Build history of the part. All positions in model axes, mm. A direction names the side the tool comes from. Round coordinates to 2 decimals unless told otherwise and drop trailing zeros. Loops run counter-clockwise (first coordinate to the right, second up) from the corner with the lowest first, then second, coordinate; pieces in that order, holes last. Notation, with made-up numbers: (41, -8) - (45, -8) arc R23 cw to (45, 10) - close; hole circle Ø3 at (-26, 75.25). An arc over 180 degrees is marked (long way). Use one line per item in the form item = value. Start each with the question number.
Q1. Drill centre lines: line 1 (Y direction, x = 0, z = 6); line 2 (Y direction, x = 28, z = 2.5); line 3 (Y direction, x = 4.5, z = 9.25). Where is each one in solid material? Low to high.
Q2. Saw through at C-C (z = 4). Count the separate pieces of the cut face and the enclosed holes in it, then the cut area to 3 significant figures.
Q3. Mould opens along X. For faces 3 (the face through (-27.44, 26.27, 5.07)), 4 (the face through (47.69, 15.02, 4.93)), 5 (the face through (9, -17, 10)) say: released by +X, released by -X, zero draft, split by the parting line, or undercut.
Q4. 3-axis set-ups, long thin cutter, end or side, ignore diameter. For faces 1 (the face through (-7, -20, 8)), 2 (the face through (8.767, -16.856, 4.93)): which of +Z, -Z, +X, -X, +Y, -Y reach the whole face in a straight line?
Q5. Saw through at A-A (x = 0). Give the cut face in (y, z).
Q6. Pin check, flat tips, straight feed: pin 1 (1 mm diameter, centred on x = -21, z = 2.5, fed in from -Y); pin 2 (2 mm diameter, centred on y = -24.5, z = 2, fed in from -X); pin 3 (2 mm diameter, centred on x = 15.5, z = 1, fed in from -Y). Stop position of each tip, or through.
Q7. Saw through at D-D (x = -23). Give the cut face in (y, z).
```python
from build123d import *

# Parameters (mm, degrees)
CROQUIS1_R              = 50
CROQUIS1_R_2            = 19
SALIENTE_EXTRUIR1_DEPTH = 10
CROQUIS4_R              = 30
CROQUIS4_R_2            = 20.75
CORTAR_EXTRUIR1_DEPTH   = 2
CROQUIS5_R              = 2.75
CORTAR_EXTRUIR2_DEPTH   = 10


with BuildPart() as part:
    # Croquis1 → Saliente-Extruir1 (new body)
    with BuildSketch(Plane.XY):
        Circle(CROQUIS1_R)
        Circle(CROQUIS1_R_2, mode=Mode.SUBTRACT)
    extrude(amount=SALIENTE_EXTRUIR1_DEPTH)

    # Croquis4 → Cortar-Extruir1 (cut)
    with BuildSketch(Plane.XY.offset(10)):
        Circle(CROQUIS4_R)
        Circle(CROQUIS4_R_2, mode=Mode.SUBTRACT)
    extrude(amount=-CORTAR_EXTRUIR1_DEPTH, mode=Mode.SUBTRACT)

    # Croquis5 → Cortar-Extruir2 (cut)
    with BuildSketch(Plane.XY.offset(10)):
        with Locations((40.602997929, 0)):
            Circle(CROQUIS5_R)
        with Locations((28.710655172, -28.710655172)):
            Circle(CROQUIS5_R)
        with Locations((0, -40.602997929)):
            Circle(CROQUIS5_R)
        with Locations((-28.710655172, -28.710655172)):
            Circle(CROQUIS5_R)
        with Locations((-40.602997929, 0)):
            Circle(CROQUIS5_R)
        with Locations((-28.710655172, 28.710655172)):
            Circle(CROQUIS5_R)
        with Locations((0, 40.602997929)):
            Circle(CROQUIS5_R)
        with Locations((28.710655172, 28.710655172)):
            Circle(CROQUIS5_R)
    extrude(amount=-CORTAR_EXTRUIR2_DEPTH, mode=Mode.SUBTRACT)


solid = part.part
```
Report:
q1.line_1 = -50 to -43.35, -37.85 to -19, 19 to 37.85, 43.35 to 50
q1.line_2 = -41.42 to -31.37, -26.05 to 26.05, 31.37 to 41.42
q1.line_3 = -49.8 to -29.66, -20.26 to -18.46, 18.46 to 20.26, 29.66 to 49.8
q2.separate_pieces = 1
q2.enclosed_holes = 9
q2.area = 6,530 mm²
q3.face_3 = undercut
q3.face_4 = split by the parting line
q3.face_5 = zero draft
q4.face_1 = +Z
q4.face_2 = +Z, -Z
q5.outline = (-50, 0) - (-43.35, 0) - (-43.35, 10) - (-50, 10) - close; (-37.85, 0) - (-19, 0) - (-19, 10) - (-20.75, 10) - (-20.75, 8) - (-30, 8) - (-30, 10) - (-37.85, 10) - close; (19, 0) - (37.85, 0) - (37.85, 10) - (30, 10) - (30, 8) - (20.75, 8) - (20.75, 10) - (19, 10) - close; (43.35, 0) - (50, 0) - (50, 10) - (43.35, 10) - close
q6.pin_1 = -45.6
q6.pin_2 = -44.13
q6.pin_3 = -47.85
q7.outline = (-44.4, 0) - (44.4, 0) - (44.4, 10) - (19.26, 10) - (19.26, 8) - (-19.26, 8) - (-19.26, 10) - (-44.4, 10) - close
